Design review of the part built by this model. Coordinates are the model's own, in mm. A direction names the side the tool comes from. Coordinates: 2 decimals unless noted, no trailing zeros. Write each loop counter-clockwise with the first axis right and the second up, starting at its lowest first coordinate (ties: lowest second). Pieces come first, ordered by that corner, then holes.
Q1. For probe 1 along Y at (x, z) = (8, -32); probe 2 along X at (y, z) = (3.5, -111); probe 3 along Z at (x, y) = (-5, -95), list the stretches that pass through material, from the lowest coordinate up.
Q2. Machinability: for faces 3 (the flat face through (7.611, -2, -71)), 4 (the cylindrical face through (8.625, -1.245, -35.002)), 5 (the flat face through (22, -2, -140)), which of the approach directions +Z, -Z, +X, -X, +Y, -Y give a long, thin tool a straight path to every point of the face, cutting with its end or side? Answer none if there is none.
Q3. Take a section at A-A (z = -32). Give the boundary of the cut face in (x, y), and give its area (3 significant figures).
Q4. Insertion check: pin 1 (3.5 mm diameter, centred on x = 8.5, z = -63, fed in from +Y); pin 2 (1 mm diameter, centred on x = 8.5, z = -140.5, fed in from -Y); pin 3 (0.6 mm diameter, centred on x = 8.5, y = 103, fed in from +Z); pin 4 (9 mm diameter, centred on x = 1.61, y = -147.5, fed in from +Z). Each pin has a flat end and moves straight along its axis. Give the tip position at first contact, or say it passes through.
Q5. Take a section at B-B (y = -100). Give the boundary of the cut face in (x, z), and give its area (3 significant figures).
Q6. Take a section at D-D (z = -96.5). Give the boundary of the cut face in (x, y).
Q7. Take a section at C-C (y = 147.5). Give the boundary of the cut face in (x, z).
Q8. Mouldability with a two-part tool opening along Y and no side actions: class faces 1 (the flat face through (9.611, -2, -73)), 2 (the cylindrical face through (26.53, -152.38, 0.99)) as pulls with the +Y half, pulls with the -Y half, needs draft (parallel to the pull), parting line crosses it, or undercut.
```python
from build123d import *

# Parameters (mm, degrees)
SKETCH_1_R          = 5
EXTRUDE_1_DEPTH     = 2
SKETCH_2_W          = 2
SKETCH_2_H          = 250
EXTRUDE_2_DEPTH     = 144
SKETCH_3_W          = 2
SKETCH_3_H          = 228
EXTRUDE_3_DEPTH     = 23
SKETCH_4_W          = 4.5
SKETCH_4_H          = 2
CUT_EXTRUDE_1_DEPTH = 2
SKETCH_5_W          = 4.5
SKETCH_5_H          = 2
CUT_EXTRUDE_2_DEPTH = 2
FILLET_3_R          = 2
FILLET_4_R          = 4
SKETCH_6_R          = 1.6
SKETCH_6_R_2        = 1.5
SKETCH_6_R_3        = 1.75
CUT_EXTRUDE_3_DEPTH = 2
CHAMFER_1_SIZE      = 1.3
SKETCH_8_R          = 3.25
SKETCH_8_R_2        = 1.1
SKETCH_8_R_3        = 1.6
CUT_EXTRUDE_4_DEPTH = 2


with BuildPart() as part:
    # Эскиз1 → Вытянуть1 (new body)
    with BuildSketch(Plane.XY):
        Polygon((-15.389384289, -165), (44.610615711, -165), (47.610615711, -162), (47.610615711, -130), (44.610615711, -127), (9.610615711, -127), (9.610615711, 127), (44.610615711, 127), (47.610615711, 130), (47.610615711, 162), (44.610615711, 165), (-15.389384289, 165), (-18.389384289, 162), (-18.389384289, -162), align=None)
        with Locations((1.610615711, -147.5)):
            Circle(SKETCH_1_R, mode=Mode.SUBTRACT)
        with Locations((27.610615711, -147.5)):
            Circle(SKETCH_1_R, mode=Mode.SUBTRACT)
        with Locations(Location((27.610615711, 147.5, 0), (0, 0, 180))):
            Circle(SKETCH_1_R, mode=Mode.SUBTRACT)
        with Locations(Location((1.610615711, 147.5, 0), (0, 0, 180))):
            Circle(SKETCH_1_R, mode=Mode.SUBTRACT)
    extrude(amount=EXTRUDE_1_DEPTH)

    # Эскиз2 → Вытянуть2 (add)
    with BuildSketch(Plane.XY.offset(2)):
        with Locations((8.610615711, 0)):
            Rectangle(SKETCH_2_W, SKETCH_2_H)
    extrude(amount=-EXTRUDE_2_DEPTH)

    # Эскиз3 → Вытянуть3 (add)
    with BuildSketch(Plane(origin=(9.610615711, 0, 0), x_dir=(0, 0, -1), z_dir=(1, 0, 0))):
        with Locations((141, 0)):
            Rectangle(SKETCH_3_W, SKETCH_3_H)
    extrude(amount=EXTRUDE_3_DEPTH)

    # Эскиз4 → Вырез-Вытянуть1 (cut)
    with BuildSketch(Plane.XY.offset(2)):
        with Locations((7.360615711, 126)):
            Rectangle(SKETCH_4_W, SKETCH_4_H)
        with Locations((7.360615711, -126)):
            Rectangle(SKETCH_4_W, SKETCH_4_H)
    extrude(amount=-CUT_EXTRUDE_1_DEPTH, mode=Mode.SUBTRACT)

    # Эскиз5 → Вырез-Вытянуть2 (cut)
    with BuildSketch(Plane(origin=(9.610615711, 0, 0), x_dir=(0, 0, -1), z_dir=(1, 0, 0))):
        with Locations((139.75, -115)):
            Rectangle(SKETCH_5_W, SKETCH_5_H)
        with Locations((139.75, 115)):
            Rectangle(SKETCH_5_W, SKETCH_5_H)
    extrude(amount=-CUT_EXTRUDE_2_DEPTH, mode=Mode.SUBTRACT)

    # Скругление3
    fillet_3_edges = [part.edges().sort_by_distance(p)[0] for p in [
        (9.610615711, 0, -140),
        (7.610615711, 0, 0),
    ]]
    fillet(fillet_3_edges, radius=FILLET_3_R)

    # Скругление4
    fillet_4_edges = [part.edges().sort_by_distance(p)[0] for p in [
        (7.610615711, 0, -142),
        (9.610615711, 0, 2),
    ]]
    fillet(fillet_4_edges, radius=FILLET_4_R)

    # Эскиз6 → Вырез-Вытянуть3 (cut)
    with BuildSketch(Plane(origin=(0, 0, -142), x_dir=(-1, 0, 0), z_dir=(0, 0, -1))):
        with Locations((-21.610615711, 0)):
            Circle(SKETCH_6_R)
        with Locations((-25.610615711, -106)):
            Circle(SKETCH_6_R_2)
        with Locations((-25.610615711, 106)):
            Circle(SKETCH_6_R_2)
        with Locations((-23.610615711, 44.5)):
            Circle(SKETCH_6_R_3)
        with Locations((-23.610615711, 70.5)):
            Circle(SKETCH_6_R_3)
    extrude(amount=-CUT_EXTRUDE_3_DEPTH, mode=Mode.SUBTRACT)

    # Фаска1
    chamfer_1_edges = [part.edges().sort_by_distance(p)[0] for p in [
        (27.110615711, -106, -142),
        (27.110615711, 106, -142),
    ]]
    chamfer(chamfer_1_edges, length=CHAMFER_1_SIZE)

    # Эскиз8 → Вырез-Вытянуть4 (cut)
    with BuildSketch(Plane(origin=(9.610615711, 0, 0), x_dir=(0, 0, -1), z_dir=(1, 0, 0))):
        with Locations((32, 0)):
            Circle(SKETCH_8_R)
        with Locations((32, -100)):
            Circle(SKETCH_8_R)
        with Locations(Location((32, 100, 0), (0, 0, 180))):
            Circle(SKETCH_8_R)
        with Locations(Location((112, 105, 0), (0, 0, 180))):
            Circle(SKETCH_8_R_2)
        with Locations(Location((72, 105, 0), (0, 0, 180))):
            Circle(SKETCH_8_R_2)
        with Locations(Location((58, 105, 0), (0, 0, 180))):
            Circle(SKETCH_8_R_3)
        with BuildLine():
            Line((80.5, 95), (103.5, 95))
            ThreePointArc((103.5, 95), (105.267766953, 95.732233047), (106, 97.5))
            Line((106, 97.5), (106, 112.5))
            ThreePointArc((106, 112.5), (105.267766953, 114.267766953), (103.5, 115))
            Line((103.5, 115), (80.5, 115))
            ThreePointArc((80.5, 115), (78.732233047, 114.267766953), (78, 112.5))
            Line((78, 112.5), (78, 97.5))
            ThreePointArc((78, 97.5), (78.732233047, 95.732233047), (80.5, 95))
        make_face()
    extrude(amount=-CUT_EXTRUDE_4_DEPTH, mode=Mode.SUBTRACT)


solid = part.part
```
Response:
1. probe 1: y = -125 to -103.25, -96.75 to -3.25, 3.25 to 96.75, 103.25 to 125
1. probe 2: x = 7.61 to 9.61
1. probe 3: z = 0 to 2
2. face 3: -Z, -X, +Y, -Y
2. face 4: +X, -X
2. face 5: +Z, +X, +Y, -Y
3. outline: (7.61, -125) - (9.61, -125) - (9.61, -103.25) - (7.61, -103.25) - close; (7.61, -96.75) - (9.61, -96.75) - (9.61, -3.25) - (7.61, -3.25) - close; (7.61, 3.25) - (9.61, 3.25) - (9.61, 96.75) - (7.61, 96.75) - close; (7.61, 103.25) - (9.61, 103.25) - (9.61, 125) - (7.61, 125) - close
3. area: 461 mm2
4. pin 1: stops at y = 125
4. pin 2: stops at y = -125
4. pin 3: stops at z = 1.05
4. pin 4: passes through
5. outline: (-18.39, 0) - (5.61, 0) arc R2 cw to (7.61, -2) - (7.61, -28.75) - (9.61, -28.75) - (9.61, -2) arc R4 ccw to (5.61, 2) - (-18.39, 2) - close; (7.61, -138) arc R4 ccw to (11.61, -142) - (32.61, -142) - (32.61, -140) - (11.61, -140) arc R2 cw to (9.61, -138) - (9.61, -35.25) - (7.61, -35.25) - close
5. area: 368 mm2
6. outline: (7.61, -125) - (9.61, -125) - (9.61, 95) - (7.61, 95) - close; (7.61, 115) - (9.61, 115) - (9.61, 125) - (7.61, 125) - close
7. outline: (-18.39, 0) - (-3.39, 0) - (-3.39, 2) - (-18.39, 2) - close; (6.61, 0) - (22.61, 0) - (22.61, 2) - (6.61, 2) - close; (32.61, 0) - (47.61, 0) - (47.61, 2) - (32.61, 2) - close
8. face 1: needs draft
8. face 2: undercut
